```python
from build123d import *

# Parameters (mm, degrees)
SKETCH_1_R      = 13.8
SKETCH_1_R_2    = 1.25
EXTRUDE_1_DEPTH = 4.6
SKETCH_2_R      = 13.8
EXTRUDE_2_DEPTH = 18.5
FILLET_1_R      = 2
CHAMFER_1_SIZE  = 2


with BuildPart() as part:
    # 草圖1 → 填料-伸長1 (new body)
    with BuildSketch(Plane(origin=(0, 0, 0), x_dir=(1, 0, 0), z_dir=(0, 1, 0))):
        with Locations(Location((0, 0, 0), (0, 0, 270))):
            Circle(SKETCH_1_R)
        with Locations(Location((0, 9.5, 0), (0, 0, 270))):
            Circle(SKETCH_1_R_2, mode=Mode.SUBTRACT)
        with Locations(Location((0, -9.5, 0), (0, 0, 270))):
            Circle(SKETCH_1_R_2, mode=Mode.SUBTRACT)
        with Locations(Location((8, 0, 0), (0, 0, 270))):
            Circle(SKETCH_1_R_2, mode=Mode.SUBTRACT)
        with Locations(Location((-8, 0, 0), (0, 0, 270))):
            Circle(SKETCH_1_R_2, mode=Mode.SUBTRACT)
    extrude(amount=EXTRUDE_1_DEPTH)

    # 草圖2 → 填料-伸長2 (add)
    with BuildSketch(Plane(origin=(0, 4.6, 0), x_dir=(1, 0, 0), z_dir=(0, 1, 0))):
        with Locations(Location((0, 0, 0), (0, 0, 270))):
            Circle(SKETCH_2_R)
    extrude(amount=EXTRUDE_2_DEPTH)

    # 圓角1
    fillet_1_edges = [part.edges().sort_by_distance(p)[0] for p in [
        (0, 23.1, -13.8),
    ]]
    fillet(fillet_1_edges, radius=FILLET_1_R)

    # 草圖5 → 旋轉1 (revolve)
    with BuildSketch(Plane.XY, mode=Mode.PRIVATE) as revolve_1_sk:
        with BuildLine():
            Line((0, 23.1), (0, 55.6))
            add(Edge.make_bspline(
                [(0, 55.6), (-0.448143347, 55.484061035), (-1.523316828, 55.079878449), (-4.652306248, 49.57128747), (-6.4, 43.797195066), (-6.4, 41.6)],
                knots=[0, 0, 0, 0, 0.157070914, 0.257070914, 1, 1, 1, 1], degree=3))
            Line((-6.4, 41.6), (-3, 41.6))
            Line((-3, 41.6), (-3, 34.6))
            Line((-3, 34.6), (-5.65, 34.6))
            Line((-5.65, 34.6), (-5.65, 25.6))
            Line((-5.65, 25.6), (-1.5, 25.6))
            Line((-1.5, 25.6), (-1.5, 23.1))
            Line((-1.5, 23.1), (0, 23.1))
        make_face()
    revolve(revolve_1_sk.sketch.rotate(Axis((0, 23.1, 0), (0, 1, 0)), 180), axis=Axis((0, 23.1, 0), (0, 1, 0)))

    # 導角1
    chamfer_1_edges = [part.edges().sort_by_distance(p)[0] for p in [
        (0, 0, -13.8),
    ]]
    chamfer(chamfer_1_edges, length=CHAMFER_1_SIZE)


solid = part.part
```
Design review of the part built by this model. Coordinates are the model's own, in mm. A direction names the side the tool comes from. Round coordinates to 2 decimals unless told otherwise and drop trailing zeros. Write each loop counter-clockwise with the first axis right and the second up, starting at its lowest first coordinate (ties: lowest second). Pieces come first, ordered by that corner, then holes.
Item 1: We need section A-A on y = 25. Write out the cut boundary in (x, z), and give its area (3 significant figures).
Item 2: The part is to be moulded in two halves that separate along X. For faces 1 (the flat face through (0, 4.6, 9)), 2 (the cylindrical face through (9.33, 11.42, -10.17)), 3 (the flat face through (-2, 23.1, 0)), say which applies: +X half, -X half, draft (parallel to the pull), parting line (faces both ways), or undercut.
Item 3: For probe 1 along X at (y, z) = (2.85, 0); probe 2 along X at (y, z) = (1, -9.5); probe 3 along Y at (x, z) = (7.75, 1.75), list the stretches that pass through material, from the lowest coordinate up.
Item 4: We need section B-B on y = 10. Write out the cut boundary in (x, z).
Item 5: For faces 4 (the flat face through (3, 41.6, 1)), 5 (the flat face through (8, 4.6, 0)), 6 (the flat face through (0, 0, 0)), list the 3-axis set-ups (+Z, -Z, +X, -X, +Y, -Y) from which the entire face can be reached by the end or side of a thin tool; tool diameter is ignored.
Item 6: Clearance check with flat-ended pins moving along their axes: pin 1 Ø3 at (x, z) = (0, -10) entering from -Y; pin 2 Ø8 at (x, y) = (2, 33) entering from +Z; pin 3 Ø4 at (x, y) = (5, 13.5) entering from -Z; pin 4 Ø5 at (x, z) = (-6, -11) entering from +Y. State where each tip first meets the part, or that it passes through.
Returned:
1. outline: circle Ø3 at (0, 0)
1. area: 7.07 mm2
2. face 1: undercut
2. face 2: parting line
2. face 3: draft
3. probe 1: x = -13.8 to -9.25, -6.75 to 6.75, 9.25 to 13.8
3. probe 2: x = -8.58 to -1.25, 1.25 to 8.58
3. probe 3: y = 0 to 23.1
4. outline: circle Ø27.6 at (0, 0)
5. face 4: none
5. face 5: -Y
5. face 6: +Z, -Z, +X, -X, -Y
6. pin 1: stops at y = 0
6. pin 2: stops at z = 5.65
6. pin 3: stops at z = -13.47
6. pin 4: stops at y = 23.1
